Source: three-view drawing plus pictorial views. Frame: mm from the lowest corner of the part. Give positions to 0.01 mm unless a question says otherwise; leave off trailing zeros. Order: outer loops, then holes, each group sorted by start corner. A loop starts at its lowest first (then second) coordinate and runs counter-clockwise, first axis right, second up. Notation, with made-up numbers: M 52.5,85.25 L 76.5,85.25 A16 cw 76.5,89.25 Z; hole C 60.5,21 d5. An arc over 180 degrees is marked long. One line per item, written item: value. Start each with the question number.
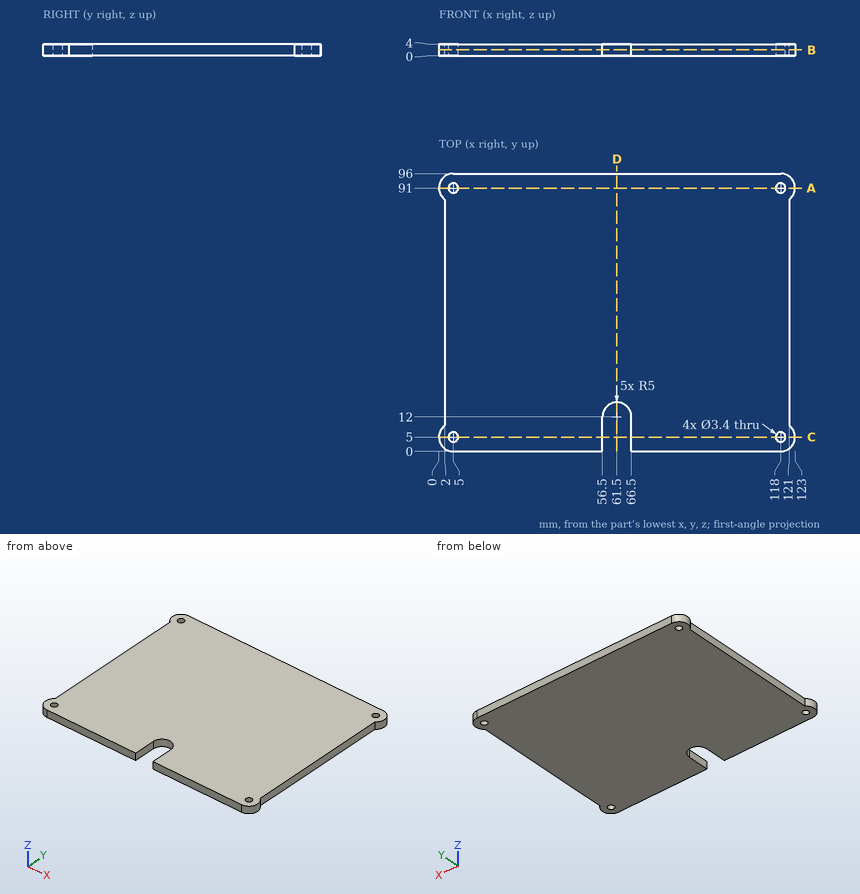
Q1. Section query D-D on x = 61.5. Return loops of the section in (y, z).
Q2. Section query A-A on y = 91. Return loops of the section in (x, z).
Q3. Section query C-C on y = 5. Return loops of the section in (x, z), and give its area (3 significant figures).
Q4. Section query B-B on z = 1.95. Return loops of the section in (x, y), and give its area (3 significant figures).
Q5. Contact query for flat-ended pins moving along their axis: pin 1 (1.2 mm diameter, centred on y = 8, z = 2.5, fed in from +X); pin 2 (2 mm diameter, centred on y = 6.5, z = 1, fed in from -X); pin 3 (2 mm diameter, centred on y = 31.5, z = 2, fed in from +X). Output: stop coordinate, or through.
Q6. Ray query, line 1 along Y through (x, z) = (116.5, 1.9); line 2 along X through (y, z) = (28, 1.25); line 3 along Y through (x, z) = (61, 3.55). Return the intervals inside material, ascending. Write a range as [from, to].
Results below:
1. outline: M 17,0 L 96,0 L 96,4 L 17,4 Z
2. outline: M 0,0 L 3.3,0 L 3.3,4 L 0,4 Z; M 6.7,0 L 116.3,0 L 116.3,4 L 6.7,4 Z; M 119.7,0 L 123,0 L 123,4 L 119.7,4 Z
3. outline: M 0,0 L 3.3,0 L 3.3,4 L 0,4 Z; M 6.7,0 L 56.5,0 L 56.5,4 L 6.7,4 Z; M 66.5,0 L 116.3,0 L 116.3,4 L 66.5,4 Z; M 119.7,0 L 123,0 L 123,4 L 119.7,4 Z
3. area: 425 mm2
4. outline: M 2,9 A5 ccw 5,0 L 56.5,0 L 56.5,12 A5 cw 66.5,12 L 66.5,0 L 118,0 A5 ccw 121,9 L 121,87 A5 ccw 118,96 L 5,96 A5 ccw 2,87 Z; hole C 5,5 d3.4; hole C 5,91 d3.4; hole C 118,5 d3.4; hole C 118,91 d3.4
4. area: 11,300 mm2
5. pin 1: x = 122.39
5. pin 2: x = 0.03
5. pin 3: x = 121
6. line 1: [0, 4.2], [5.8, 90.2], [91.8, 96]
6. line 2: [2, 121]
6. line 3: [16.97, 96]
